from build123d import *

# Parameters (mm, degrees)
BOSS_EXTRUDE1_DEPTH = 519.5
FILLET1_R           = 15
SKETCH2_W           = 33
SKETCH2_H           = 202
CUT_EXTRUDE1_DEPTH  = 57.9350001
FILLET2_R           = 10


with BuildPart() as part:
    # Sketch1 → Boss-Extrude1 (new body, symmetric)
    with BuildSketch(Plane.XY):
        with BuildLine():
            Line((40.754430434, 5), (56.51128828, 6.933146615))
            ThreePointArc((56.51128828, 6.933146615), (0, 56.935), (-56.51128828, 6.933146615))
            Line((-56.51128828, 6.933146615), (-40.754430434, 5))
            ThreePointArc((-40.754430434, 5), (0, 41.06), (40.754430434, 5))
        make_face()
    extrude(amount=BOSS_EXTRUDE1_DEPTH, both=True)

    # Fillet1
    fillet1_edges = [part.edges().sort_by_distance(p)[0] for p in [
        (-48.632859357, 5.966573307, 519.5),
        (-48.632859357, 5.966573307, -519.5),
        (48.632859357, 5.966573307, -519.5),
        (48.632859357, 5.966573307, 519.5),
    ]]
    fillet(fillet1_edges, radius=FILLET1_R)

    # Sketch2 → Cut-Extrude1 (cut, through all)
    with BuildSketch(Plane(origin=(0, 0, 0), x_dir=(1, 0, 0), z_dir=(0, 1, 0))):
        with Locations((0, -163)):
            Rectangle(SKETCH2_W, SKETCH2_H)
    extrude(amount=CUT_EXTRUDE1_DEPTH, mode=Mode.SUBTRACT)

    # Fillet2
    fillet2_edges = [part.edges().sort_by_distance(p)[0] for p in [
        (-16.5, 46.045270275, 62),
        (-16.5, 46.045270275, 264),
        (16.5, 46.045270275, 264),
        (16.5, 46.045270275, 62),
    ]]
    fillet(fillet2_edges, radius=FILLET2_R)


solid = part.part
Could you check a few things on this model? Use its own coordinates, in mm. A direction names the side the tool comes from. Give positions to 0.01 mm unless a question says otherwise; leave off trailing zeros. Order: outer loops, then holes, each group sorted by start corner. A loop starts at its lowest first (then second) coordinate and runs counter-clockwise, first axis right, second up.
1. Suppose I cut it at D-D (x = 25). Write out the boundary of the cut face in (y, z), plus the area to 3 significant figures.
Answers below:
outline: (32.57, -519.5) - (51.15, -519.5) - (51.15, 519.5) - (32.57, 519.5) - close
area: 19,300 mm2
2. Suppose I cut it at C-C (z = -278). Write out the boundary of the cut face in (x, y) (3 decimals), plus the area to 3 significant figures.
Answers below:
outline: (-56.511, 6.933) - (-40.754, 5) arc R41.06 cw to (40.754, 5) - (56.511, 6.933) arc R56.935 ccw to start
area: 2,250 mm2
3. Which directions (+Z, -Z, +X, -X, +Y, -Y) give clear straight access to the entire face, cutting with the end or side of a thin tool? Please do faces 5 (the flat face through (16.5, 46, 164)), 6 (the flat face through (48.523, 5.953, 7.063)).
Answers below:
face 5: +Y, -Y
face 6: +Z, -Z, +X, -Y
4. For pin 1 (8.5 mm diameter, centred on y = 48.5, z = 140, fed in from -X); pin 2 (3 mm diameter, centred on y = 42.5, z = 43.5, fed in from -X); pin 3 (6 mm diameter, centred on y = 29.5, z = -336.5, fed in from -X), each with a flat end and sliding along its axis, tell me the tip position at first contact or that it passes through.
Answers below:
pin 1: stops at x = -35.83
pin 2: stops at x = -39.5
pin 3: stops at x = -50.39
5. I need wall thicknesses on L1, parallel to X at y = 9, z = 383.5; L2, parallel to X at y = 44, z = -111; L3, parallel to X at y = 27.5, z = -395. Which ranges of each line are inside material? Lowest first, please.
Answers below:
L1: x = -56.22 to -40.06, 40.06 to 56.22
L2: x = -36.13 to 36.13
L3: x = -49.85 to -30.49, 30.49 to 49.85
6. Suppose I cut it at B-B (y = 29.5). Write out the boundary of the cut face in (x, z).
Answers below:
outline: (-48.7, -519.5) - (-28.56, -519.5) - (-28.56, 519.5) - (-48.7, 519.5) - close; (28.56, -519.5) - (48.7, -519.5) - (48.7, 519.5) - (28.56, 519.5) - close
7. Thinking about a two-plate mould opening in X: for faces 1 (the cylindrical face through (-0.83, 41.05, 7.27)), 2 (the cylindrical face through (1.155, 56.923, 7.273)), 3 (the flat face through (-48.74, 5.98, 7.06)), 4 (the flat face through (-1, 43, 519.5)), which applies, +X half, -X half, draft (parallel to the pull), parting line (faces both ways), or undercut?
Answers below:
face 1: undercut
face 2: parting line
face 3: -X half
face 4: draft
8. Suppose I cut it at A-A (z = 127). Write out the boundary of the cut face in (x, y) (3 decimals), plus the area to 3 significant figures.
Answers below:
outline: (-56.511, 6.933) - (-40.754, 5) arc R41.06 cw to (-16.5, 37.599) - (-16.5, 54.492) arc R56.935 ccw to start; (16.5, 37.599) arc R41.06 cw to (40.754, 5) - (56.511, 6.933) arc R56.935 ccw to (16.5, 54.492) - close
area: 1,720 mm2
